Geometry check sheet. Reference: drawing and pictorial views, mm from the part's lowest x, y, z. Give positions to 0.01 mm unless a question says otherwise; leave off trailing zeros. Loops run counter-clockwise (first coordinate to the right, second up) from the corner with the lowest first, then second, coordinate; pieces in that order, holes last. Notation, with made-up numbers: (33, 18.25) -> (39, 18.25) arc R15 ccw to (39, 43.25) -> close; hole circle Ø1 at (-33, 31.25). An arc over 180 degrees is marked (long way). Write item = value, one per line. Start each with the question number.
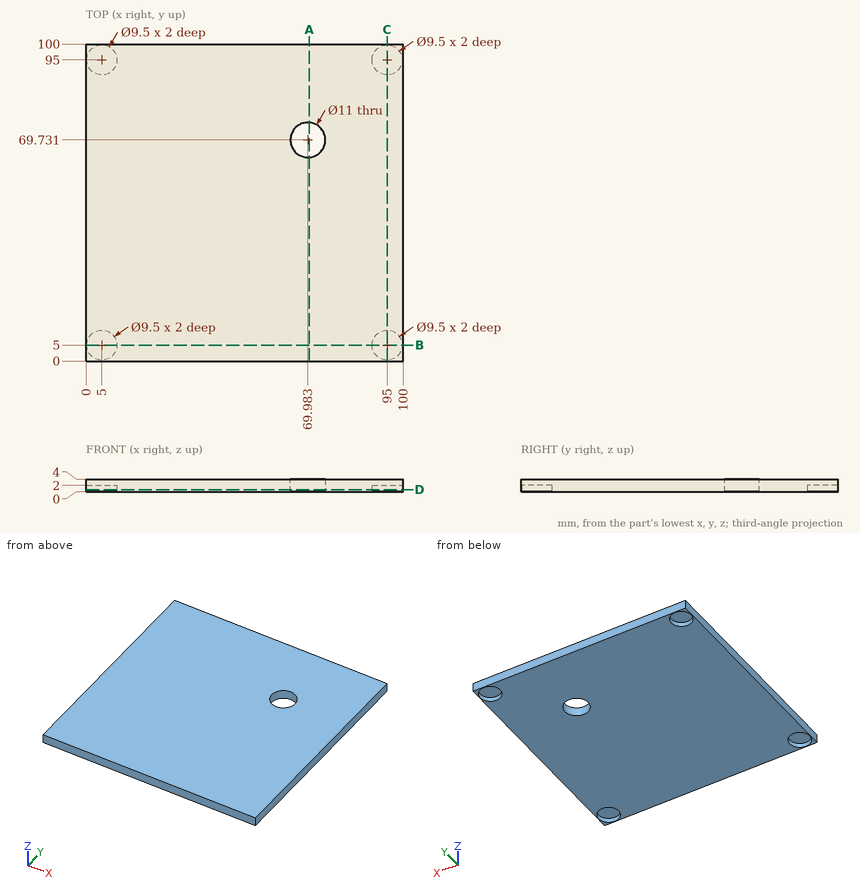
1) Section check D-D (z = 0.65). Enter the section's corners in (x, y).
2) Section check A-A (x = 70.5). Enter the section's corners in (y, z) (1 decimal).
3) Section check B-B (y = 5). Enter the section's corners in (x, z).
4) Depth check by flat-ended pin: pin 1 Ø2 at (x, y) = (31, 51) entering from -Z; pin 2 Ø3 at (x, y) = (96, 96.5) entering from -Z; pin 3 Ø6.5 at (x, y) = (69.98, 69.73) entering from -Z. Enter the tip coordinate at first touch or a pass-through.
5) Thickness scan on line 1 (Y direction, x = 95, z = 1.25); line 2 (Y direction, x = 68, z = 3.85); line 3 (Y direction, x = 66.5, z = 0.35) (1 decimal). Record the ranges inside material, lowest first.
Check result:
q1.outline = (0, 0) -> (100, 0) -> (100, 100) -> (0, 100) -> close; hole circle Ø9.5 at (5, 5); hole circle Ø9.5 at (5, 95); hole circle Ø11 at (69.98, 69.73); hole circle Ø9.5 at (95, 5); hole circle Ø9.5 at (95, 95)
q2.outline = (0, 0) -> (64.3, 0) -> (64.3, 4) -> (0, 4) -> close; (75.2, 0) -> (100, 0) -> (100, 4) -> (75.2, 4) -> close
q3.outline = (0, 0) -> (0.25, 0) -> (0.25, 2) -> (9.75, 2) -> (9.75, 0) -> (90.25, 0) -> (90.25, 2) -> (99.75, 2) -> (99.75, 0) -> (100, 0) -> (100, 4) -> (0, 4) -> close
q4.pin_1 = 0
q4.pin_2 = 2
q4.pin_3 = through
q5.line_1 = 0 to 0.25, 9.75 to 90.25, 99.75 to 100
q5.line_2 = 0 to 64.6, 74.86 to 100
q5.line_3 = 0 to 65.5, 74 to 100
